Check sheet for the modelled part. Datum: model origin and axes. Units: mm. A direction names the side the tool comes from. Give positions to 0.01 mm unless a question says otherwise; leave off trailing zeros. Loops run counter-clockwise (first coordinate to the right, second up) from the corner with the lowest first, then second, coordinate; pieces in that order, holes last. Notation, with made-up numbers: (45.25, 57.25) -> (100.25, 57.25) arc R35 cw to (100.25, 92.25) -> close; hole circle Ø8 at (50, 54.5). An arc over 180 degrees is marked (long way). Write each question's results on one line, items separated by ' | '. Start each with the question number.
1. Cross-section at A-A on z = -12.7. Record the boundary of the cut face in (x, y), and give its area (3 significant figures).
2. Mould release check, pull along Z, two halves, no side actions. Record for faces 1 (the face through (38, 13, 0)), 2 (the face through (4.378, 4.559, -7.282)), 3 (the face through (38, 0, -7)), 4 (the face through (4.378, 19.139, -17.033)): +Z half, -Z half, draft (parallel to the pull), parting line (faces both ways), or undercut.
3. Tool access check on faces 5 (the face through (4.378, 17.259, -7.282)), 6 (the face through (72.33, 5.577, -17.185)), 7 (the face through (38, 13, -25.4)). Record the directions out of +Z, -Z, +X, -X, +Y, -Y that give a thin tool (end or side, any length) a straight path to the whole face; none if there is none.
4. Cross-section at C-C on x = 71.5. Record the boundary of the cut face in (y, z).
5. Cross-section at B-B on y = 2.5. Record the boundary of the cut face in (x, z), and give its area (3 significant figures).
6. Gauge pin test, flat end, axial feed: pin 1 Ø2.5 at (y, z) = (19.05, -6.35) entering from +X. Record the tip position at first contact, or that the pin passes through.
7. Material ranges on L1, parallel to Z at x = 71, y = 19.05; L2, parallel to Y at x = 74.5, z = -19.05; L3, parallel to X at y = 20.25, z = -12.75, recorded low to high. Write a range as from..to.
from build123d import *

# Parameters (mm, degrees)
SKETCH1_W                  = 76.708
SKETCH1_H                  = 25.4
BOSS_EXTRUDE1_DEPTH        = 25.4
F_10_32_TAPPED_HOLE1_D     = 4.0386
F_10_32_TAPPED_HOLE1_DEPTH = 8.636
F_10_32_TAPPED_HOLE1_TIP   = 1.213317848
F_10_32_TAPPED_HOLE2_D     = 4.0386
F_10_32_TAPPED_HOLE2_DEPTH = 8.636
F_10_32_TAPPED_HOLE2_TIP   = 1.213317848
F_6_0MM_DOWEL_HOLE1_D      = 7


with BuildPart() as part:
    # Sketch1 → Boss-Extrude1 (new body)
    with BuildSketch(Plane(origin=(0, 0, 0), x_dir=(1, 0, 0), z_dir=(0, 1, 0))):
        with Locations((38.354, 12.7)):
            Rectangle(SKETCH1_W, SKETCH1_H)
    extrude(amount=BOSS_EXTRUDE1_DEPTH)

    # #10-32 Tapped Hole1
    with Locations(Plane(origin=(76.708, 0, 0), x_dir=(0, 0, -1), z_dir=(1, 0, 0))):
        with Locations((6.35, 19.05), (19.05, 19.05), (19.05, 6.35), (6.35, 6.35)):
            Hole(F_10_32_TAPPED_HOLE1_D / 2, depth=F_10_32_TAPPED_HOLE1_DEPTH)
            with Locations((0, 0, -(F_10_32_TAPPED_HOLE1_DEPTH + F_10_32_TAPPED_HOLE1_TIP / 2))):  # 118° drill point
                Cone(0, F_10_32_TAPPED_HOLE1_D / 2, F_10_32_TAPPED_HOLE1_TIP, mode=Mode.SUBTRACT)

    # #10-32 Tapped Hole2
    with Locations(Plane.ZY):
        with Locations((-19.05, 19.05), (-6.35, 19.05), (-6.35, 6.35), (-19.05, 6.35)):
            Hole(F_10_32_TAPPED_HOLE2_D / 2, depth=F_10_32_TAPPED_HOLE2_DEPTH)
            with Locations((0, 0, -(F_10_32_TAPPED_HOLE2_DEPTH + F_10_32_TAPPED_HOLE2_TIP / 2))):  # 118° drill point
                Cone(0, F_10_32_TAPPED_HOLE2_D / 2, F_10_32_TAPPED_HOLE2_TIP, mode=Mode.SUBTRACT)

    # Ø6.0mm Dowel Hole1 (through all)
    with Locations(Plane(origin=(0, 25.4, 0), x_dir=(1, 0, 0), z_dir=(0, 1, 0))):
        with Locations((38.354, 12.7)):
            Hole(F_6_0MM_DOWEL_HOLE1_D / 2)


solid = part.part
Geometry says:
1) outline: (0, 0) -> (34.85, 0) -> (34.85, 25.4) -> (0, 25.4) -> close; (41.85, 0) -> (76.71, 0) -> (76.71, 25.4) -> (41.85, 25.4) -> close | area: 1,770 mm^2
2) face 1: +Z half | face 2: undercut | face 3: draft | face 4: undercut
3) face 5: -X | face 6: +X | face 7: -Z, +X, -X, +Y, -Y
4) outline: (0, -25.4) -> (25.4, -25.4) -> (25.4, 0) -> (0, 0) -> close; hole circle Ø4.04 at (6.35, -19.05); hole circle Ø4.04 at (6.35, -6.35); hole circle Ø4.04 at (19.05, -19.05); hole circle Ø4.04 at (19.05, -6.35)
5) outline: (0, -25.4) -> (76.71, -25.4) -> (76.71, 0) -> (0, 0) -> close; hole circle Ø7 at (38.35, -12.7) | area: 1,910 mm^2
6) pin 1: x = 67.61
7) L1: -25.4..-21.07, -17.03..-8.37, -4.33..0 | L2: 0..4.33, 8.37..17.03, 21.07..25.4 | L3: 0..34.85, 41.85..76.71
